Check sheet for the modelled part. Datum: model origin and axes. Units: mm. Face numbers are marked on the shaded views. A direction names the side the tool comes from. Round coordinates to 2 decimals unless told otherwise and drop trailing zeros. Order: outer loops, then holes, each group sorted by start corner. A loop starts at its lowest first (then second) coordinate and runs counter-clockwise, first axis right, second up. Notation, with made-up numbers: (-17.5, 7) -> (-0.5, 7) arc R24 ccw to (-0.5, 42) -> close; hole circle Ø1 at (43.25, -28.5). An arc over 180 degrees is marked (long way). Use CSV: the item, a comma, the result in double quotes.
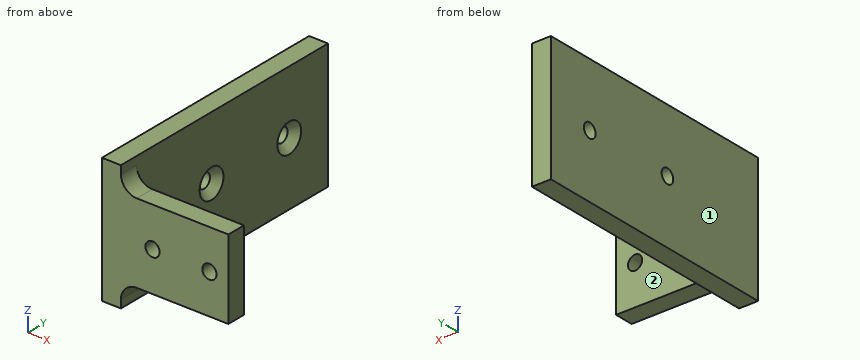
Autodesk Inventor part; units mm, degrees
ref_plane "YZ Plane" through (0, 0, 0) normal (1, 0, 0) x (0, 1, 0)
ref_plane "XZ Plane" through (0, 0, 0) normal (0, 1, 0) x (-1, 0, 0)
ref_plane "XY Plane" through (0, 0, 0) normal (0, 0, 1) x (1, 0, 0)
sketch "Skizze1" plane through (0, 0, 0) normal (0, 0, 1) x (1, 0, 0)
  line L0 (0, 0) -> (2.7641, 0)
  line L1 (6, 6) -> (6, 80)
  line L2 (6, 80) -> (0, 80)
  line L3 (0, 80) -> (0, 0)
  line L4 (-8, 0) -> (48, 0)
  line L5 (0, -16) -> (0, 96)
  line L6 (0, 0) -> (40, 0)
  line L7 (40, 0) -> (40, 6)
  line L8 (40, 6) -> (6, 6)
  line L9 (0, 2.8256) -> (0, 0)
  dimension "d0" = 80
  dimension "d1" = 40
  dimension "d2" = 6
extrude "Extrusion1" add sketch "Skizze1" along normal blind 40
sketch "Skizze2" plane through (6, 6, 0) normal (0, 1, 0) x (1, 0, 0)
  line L0 (34, 0) -> (34, -40)
  line L1 (0, 0) -> (0, -40)
  line L2 (0, -20) -> (34, -20)
  line L3 (0, -7.5) -> (34, -7.5)
  line L4 (34, -7.5) -> (34, -32.5)
  line L5 (34, -32.5) -> (0, -32.5)
  line L6 (0, -32.5) -> (0, -7.5)
  line L7 (34, -7.5) -> (0, -7.5)
  line L8 (0, -7.5) -> (0, 0)
  line L9 (0, 0) -> (34, 0)
  line L10 (34, 0) -> (34, -7.5)
  line L11 (34, -40) -> (0, -40)
  line L12 (0, -40) -> (0, -32.5)
  line L13 (0, -32.5) -> (34, -32.5)
  line L14 (34, -32.5) -> (34, -40)
  point P0 (-6, 0)
  dimension "d5" = 25
extrude "Extrusion2" cut sketch "Skizze2" against normal through all contours L0 L3 L1 L9 | L0 L11 L1 L5
sketch "Skizze3" plane through (0, 0, 0) normal (-1, 0, 0) x (0, 0, 1)
  line L0 (0, 80) -> (40, 80)
  line L1 (0, 0) -> (40, 0)
  line L2 (20, 80) -> (20, 0)
  point P0 (20, 65)
  point P1 (20, 35)
  dimension "d8" = 15
  dimension "d9" = 30
hole "Bohrung1" at (0, 65, 20) at (0, 35, 20) direction (1, 0, 0) diameter 4 end through all
sketch "Skizze4" plane through (6, 6, 32.5) normal (0, 1, 0) x (1, 0, 0)
  line L0 (34, 25) -> (34, 0)
  line L1 (0, 25) -> (0, 0)
  line L2 (34, 12.5) -> (0, 12.5)
  point P0 (-6, 32.5)
  point P1 (28, 12.5)
  point P2 (10, 12.5)
  dimension "d17" = 18
  dimension "d44" = 6
hole "Bohrung2" at (34, 6, 20) at (16, 6, 20) direction (0, -1, 0) diameter 4.5 end through all
fillet "Rundung1" radius 5 2 edges at (6, 3, 32.5) (6, 3, 7.5)
sketch "Skizze5" plane through (6, 0, 0) normal (1, 0, 0) x (0, 0, -1)
  circle A0 centre (-20, 65) radius 2
  circle A1 centre (-20, 35) radius 2
hole "Bohrung5" at (6, 65, 20) at (6, 35, 20) direction (-1, 0, 0) diameter 4.5 end through all countersink diameter 9.2 countersink angle 90
properties part number "1_0204_003"
Q1. Go/stop test with flat-tipped pins: pin 1 (6 mm diameter, centred on y = 30, z = 8, fed in from -X); pin 2 (4 mm diameter, centred on y = 60.5, z = 17.5, fed in from +X); pin 3 (6.5 mm diameter, centred on x = 24.5, y = 4, fed in from -Z); pin 4 (1.8 mm diameter, centred on x = 18.5, y = 4, fed in from +Z). Record where each tip stops, or that it passes through.
Result sheet:
pin 1,"stops at x = 0"
pin 2,"stops at x = 6"
pin 3,"stops at z = 7.5"
pin 4,"stops at z = 32.5"
Q2. Sectioned sample at B-B, the plane z = 20. Enter the section's corners in (x, y).
Result sheet:
outline,"(0, 0) -> (13.75, 0) -> (13.75, 6) -> (6, 6) -> (6, 30.4) -> (3.65, 32.75) -> (0, 32.75) -> close; (0, 37.25) -> (3.65, 37.25) -> (6, 39.6) -> (6, 60.4) -> (3.65, 62.75) -> (0, 62.75) -> close; (0, 67.25) -> (3.65, 67.25) -> (6, 69.6) -> (6, 80) -> (0, 80) -> close; (18.25, 0) -> (31.75, 0) -> (31.75, 6) -> (18.25, 6) -> close; (36.25, 0) -> (40, 0) -> (40, 6) -> (36.25, 6) -> close"
Q3. Scan lines: L1, parallel to X at y = 2.25, z = 20; L2, parallel to Y at x = 2, z = 20; L3, parallel to Z at x = 0.8, y = 65. Record each from-to range of solid material in increasing order.
Result sheet:
L1,"x = 0 to 13.75, 18.25 to 31.75, 36.25 to 40"
L2,"y = 0 to 32.75, 37.25 to 62.75, 67.25 to 80"
L3,"z = 0 to 17.75, 22.25 to 40"
Q4. Access from +Z, -Z, +X, -X, +Y, -Y to the whole of each face (thin tool, end or side, straight path). Record for the marked faces 1 and 2.
Result sheet:
face 1,"+Z, -Z, -X, +Y, -Y"
face 2,"+Z, -Z, +X, +Y"
Q5. Sectioned sample at C-C, the plane y = 5. Enter the section's corners in (x, z).
Result sheet:
outline,"(0, 0) -> (6, 0) -> (6, 2.5) arc R5 cw to (11, 7.5) -> (40, 7.5) -> (40, 32.5) -> (11, 32.5) arc R5 cw to (6, 37.5) -> (6, 40) -> (0, 40) -> close; hole circle Ø4.5 at (16, 20); hole circle Ø4.5 at (34, 20)"
Q6. Sectioned sample at D-D, the plane y = 65. Enter the section's corners in (x, z).
Result sheet:
outline,"(0, 0) -> (6, 0) -> (6, 15.4) -> (3.65, 17.75) -> (0, 17.75) -> close; (0, 22.25) -> (3.65, 22.25) -> (6, 24.6) -> (6, 40) -> (0, 40) -> close"
Q7. Sectioned sample at A-A, the plane x = 34. Enter the section's corners in (y, z), then the cut area to 3 significant figures.
Result sheet:
outline,"(0, 7.5) -> (6, 7.5) -> (6, 17.75) -> (0, 17.75) -> close; (0, 22.25) -> (6, 22.25) -> (6, 32.5) -> (0, 32.5) -> close"
area,"123 mm^2"
